Part model, mm, in its own coordinate system. Face numbers are marked on the shaded views. Give positions to 0.01 mm unless a question says otherwise; leave off trailing zeros. Write each loop counter-clockwise with the first axis right and the second up, starting at its lowest first coordinate (ties: lowest second). Pieces come first, ordered by that corner, then holes. Notation, with made-up numbers: M 60,62.25 L 103,62.25 A17 ccw 103,92.25 Z; hole C 22.25,60.25 d6. An arc over 180 degrees is marked long. Use a Markdown table: item, result. Add a question column.
from build123d import *

# Parameters (mm, degrees)
SKETCH1_R           = 4.5
BOSS_EXTRUDE1_DEPTH = 3
FILLET1_R           = 1
SKETCH6_R           = 1.75
BOSS_EXTRUDE3_DEPTH = 14
BOSS_EXTRUDE4_DEPTH = 1


with BuildPart() as part:
    # Sketch1 → Boss-Extrude1 (new body)
    with BuildSketch(Plane(origin=(0, 115.601531763, -5.053e-06), x_dir=(1, 0, 0), z_dir=(0, 1, -4.4e-08))):
        with Locations((40.91030477, -143.155151275)):
            Circle(SKETCH1_R)
    extrude(amount=BOSS_EXTRUDE1_DEPTH)

    # Fillet1
    fillet1_edges = [part.edges().sort_by_distance(p)[0] for p in [
        (36.41030477, 118.601538021, 143.155146091),
    ]]
    fillet(fillet1_edges, radius=FILLET1_R)

    # Sketch6 → Boss-Extrude3 (add)
    with BuildSketch(Plane(origin=(0, 115.601531763, -5.053e-06), x_dir=(-1, 0, 0), z_dir=(0, -1, 4.4e-08))):
        with Locations((-40.91030477, -143.155151275)):
            Circle(SKETCH6_R)
    extrude(amount=BOSS_EXTRUDE3_DEPTH)

    # Sketch7 → Boss-Extrude4 (add)
    with BuildSketch(Plane(origin=(0, 118.601531763, -5.184e-06), x_dir=(1, 0, 0), z_dir=(0, 1, -4.4e-08))):
        with BuildLine():
            add(Edge.make_bspline(
                [(39.781937709, -141.764742389), (39.830929551, -141.76598327), (39.927153571, -141.768420461), (40.068573285, -141.787076688), (40.203582672, -141.81935237), (40.333281527, -141.862338077), (40.45611848, -141.91968038), (40.573018119, -141.988989986), (40.683702303, -142.070993023), (40.786679181, -142.165055594), (40.880913899, -142.267399038), (40.96393704, -142.376617458), (41.033516631, -142.492050481), (41.090655886, -142.613351228), (41.135482812, -142.740245371), (41.16641566, -142.873409408), (41.186174857, -143.011980537), (41.188484879, -143.106494893), (41.189656726, -143.154440907)],
                knots=[0, 0, 0, 0, 0.000146952, 0.000288625, 0.000426954, 0.000562883, 0.000697813, 0.000832796, 0.000969967, 0.001110296, 0.00125059, 0.001386805, 0.001521151, 0.001654161, 0.00178843, 0.001924058, 0.002063701, 0.002207476, 0.002207476, 0.002207476, 0.002207476], degree=3))
            add(Edge.make_bspline(
                [(41.189656726, -143.154440907), (41.188485051, -143.202033739), (41.186175543, -143.295844723), (41.166393194, -143.433536493), (41.135368152, -143.565896722), (41.091072165, -143.692704448), (41.034205286, -143.814093439), (40.964162388, -143.929744292), (40.88165683, -144.039694918), (40.787762365, -144.142740802), (40.685405625, -144.237232938), (40.575618459, -144.319570421), (40.460869938, -144.390421396), (40.339683432, -144.446954293), (40.213666142, -144.492139018), (40.08169022, -144.522946066), (39.944374075, -144.542817819), (39.850733494, -144.545099673), (39.803138297, -144.546259483)],
                knots=[0, 0, 0, 0, 0.000142716, 0.000281309, 0.000416421, 0.000550016, 0.000683505, 0.000817851, 0.000954912, 0.001095241, 0.001235536, 0.001372174, 0.001506342, 0.001639351, 0.001772621, 0.001907218, 0.002045287, 0.002188002, 0.002188002, 0.002188002, 0.002188002], degree=3))
            add(Edge.make_bspline(
                [(39.803138297, -144.546259483), (39.755192532, -144.545088221), (39.660678666, -144.54277935), (39.521933407, -144.522987455), (39.388675827, -144.492037779), (39.261287002, -144.447807431), (39.139695894, -144.390644406), (39.023664701, -144.320942286), (38.913659155, -144.238235697), (38.810591287, -144.144371679), (38.716286834, -144.042188423), (38.634069925, -143.932700623), (38.564352131, -143.818056319), (38.50738104, -143.697937357), (38.46227755, -143.572924422), (38.431506646, -143.442183608), (38.41159792, -143.306460291), (38.409303721, -143.214050481), (38.408139632, -143.16716126)],
                knots=[0, 0, 0, 0, 0.000143775, 0.000283418, 0.000419562, 0.000553657, 0.000687146, 0.000821946, 0.000959007, 0.001099336, 0.001239631, 0.001375527, 0.001509419, 0.001641471, 0.001773742, 0.001907308, 0.002043802, 0.0021844, 0.0021844, 0.0021844, 0.0021844], degree=3))
            add(Edge.make_bspline(
                [(38.408139632, -143.16716126), (38.408543791, -143.135688944), (38.40934701, -143.073141351), (38.419016921, -142.980260052), (38.433048683, -142.888872471), (38.453158462, -142.799238481), (38.479459306, -142.711577499), (38.510492683, -142.625284958), (38.548396019, -142.541235357), (38.59124389, -142.459030531), (38.639066804, -142.379951936), (38.691889543, -142.305203679), (38.747856756, -142.234158521), (38.809212417, -142.168657512), (38.873934373, -142.106795165), (38.943072551, -142.049522158), (39.016205081, -141.996322047), (39.093646642, -141.948379289), (39.173489029, -141.905018514), (39.255794688, -141.867809139), (39.339445787, -141.835873128), (39.424834122, -141.809988695), (39.511732943, -141.789553763), (39.600331912, -141.77563868), (39.690560442, -141.765944106), (39.75134757, -141.765144685), (39.781937709, -141.764742389)],
                knots=[0, 0, 0, 0, 9.438e-05, 0.000187569, 0.000279848, 0.000371657, 0.000462884, 0.000554264, 0.000646556, 0.00073925, 0.000832238, 0.000923551, 0.001013693, 0.001103328, 0.001192553, 0.001282131, 0.001372457, 0.00146364, 0.001555178, 0.001644836, 0.001734413, 0.00182361, 0.001912319, 0.002001981, 0.002092533, 0.002184264, 0.002184264, 0.002184264, 0.002184264], degree=3))
        make_face()
        with BuildLine():
            add(Edge.make_bspline(
                [(39.793598032, -142.036109911), (39.768489351, -142.036415989), (39.718512029, -142.037025218), (39.6442136, -142.045050193), (39.570892316, -142.056487669), (39.498533037, -142.072802271), (39.42743852, -142.095030335), (39.356946081, -142.12061245), (39.287698534, -142.151773631), (39.219924487, -142.186980378), (39.154220829, -142.225948908), (39.092223132, -142.269016851), (39.033770895, -142.31517421), (38.979007235, -142.364528706), (38.928092956, -142.417331679), (38.88002595, -142.472782628), (38.836732873, -142.532466498), (38.797056276, -142.594764841), (38.761550826, -142.659596512), (38.729978206, -142.726278968), (38.704151843, -142.795356148), (38.683089213, -142.866078636), (38.665626856, -142.938334424), (38.654564306, -143.012671643), (38.646451153, -143.088716757), (38.645876746, -143.140107802), (38.645586213, -143.16610123)],
                knots=[0, 0, 0, 0, 7.5292e-05, 0.000149864, 0.00022393, 0.000297861, 0.000372133, 0.000447257, 0.000522705, 0.000599749, 0.000676284, 0.000751707, 0.000826039, 0.000899591, 0.000972681, 0.001045978, 0.001119549, 0.001193655, 0.001267426, 0.001341167, 0.0014148, 0.001488412, 0.001562462, 0.001637575, 0.001713729, 0.00179167, 0.00179167, 0.00179167, 0.00179167], degree=3))
            add(Edge.make_bspline(
                [(38.645586213, -143.16610123), (38.646549948, -143.204323861), (38.648445913, -143.279519602), (38.66504479, -143.389713377), (38.690612592, -143.495613451), (38.728302387, -143.59664037), (38.775436483, -143.693662536), (38.833665144, -143.785819258), (38.902652667, -143.873135443), (38.981017357, -143.95500151), (39.066683927, -144.029724231), (39.15764974, -144.095313236), (39.252940265, -144.150807889), (39.352803996, -144.196017676), (39.45670779, -144.231842061), (39.565321177, -144.25639436), (39.677920631, -144.272553186), (39.754672972, -144.274104972), (39.793598032, -144.274891962)],
                knots=[0, 0, 0, 0, 0.000114606, 0.000225465, 0.000333574, 0.000440894, 0.000548272, 0.000656647, 0.000767237, 0.000881574, 0.000996152, 0.001107795, 0.001217519, 0.00132639, 0.001436175, 0.001546614, 0.001660023, 0.001776724, 0.001776724, 0.001776724, 0.001776724], degree=3))
            add(Edge.make_bspline(
                [(39.793598032, -144.274891962), (39.819761167, -144.274532503), (39.871650522, -144.273819589), (39.948829875, -144.266639042), (40.024618797, -144.255124474), (40.098910985, -144.238545942), (40.171622122, -144.217797161), (40.243055694, -144.193147272), (40.31245083, -144.162394219), (40.380682969, -144.128415708), (40.445994414, -144.089680589), (40.508341989, -144.048074369), (40.566154188, -144.001984995), (40.620876879, -143.953363791), (40.672000191, -143.901230406), (40.719178411, -143.845652619), (40.762252678, -143.786279622), (40.801914208, -143.724075774), (40.837295246, -143.659066702), (40.868122303, -143.592142481), (40.89427532, -143.523467905), (40.915387939, -143.452943919), (40.931932306, -143.380704468), (40.943332007, -143.306652825), (40.951306125, -143.230937132), (40.951907165, -143.179726003), (40.952210145, -143.153910892)],
                knots=[0, 0, 0, 0, 7.8471e-05, 0.000155631, 0.000232315, 0.000308314, 0.000383811, 0.000459075, 0.000534795, 0.000611356, 0.000687621, 0.000762445, 0.000836033, 0.000909231, 0.000981942, 0.001054895, 0.001127725, 0.001201831, 0.001276067, 0.001349584, 0.001422723, 0.001496334, 0.001570264, 0.001644854, 0.001721008, 0.001798419, 0.001798419, 0.001798419, 0.001798419], degree=3))
            add(Edge.make_bspline(
                [(40.952210145, -143.153910892), (40.951906923, -143.128272386), (40.951305425, -143.077413686), (40.943335816, -143.002226044), (40.931920262, -142.928707247), (40.915468691, -142.85714592), (40.894264111, -142.787523821), (40.868117736, -142.719906339), (40.837285992, -142.654041572), (40.801901203, -142.590092312), (40.762126146, -142.528728075), (40.718663236, -142.470064347), (40.67076205, -142.41520281), (40.619791186, -142.362789083), (40.564477481, -142.313941036), (40.505071497, -142.268642464), (40.442294431, -142.225800167), (40.375825628, -142.187151677), (40.30722752, -142.151459965), (40.236837802, -142.120880933), (40.165453899, -142.094897248), (40.093257338, -142.072735018), (40.019640444, -142.056551567), (39.945100645, -142.045039886), (39.869741068, -142.037028011), (39.819059587, -142.036416915), (39.793598032, -142.036109911)],
                knots=[0, 0, 0, 0, 7.6881e-05, 0.000152508, 0.000226574, 0.000299988, 0.000372585, 0.000444733, 0.000517289, 0.000590596, 0.000663809, 0.000736527, 0.000809423, 0.000882134, 0.000955727, 0.00103057, 0.00110613, 0.001183578, 0.001261092, 0.001337996, 0.001413617, 0.001488903, 0.001564385, 0.001639498, 0.001715125, 0.001791477, 0.001791477, 0.001791477, 0.001791477], degree=3))
        make_face(mode=Mode.SUBTRACT)
        Polygon((41.732391769, -141.83258427), (41.96983835, -141.83258427), (41.96983835, -142.840142196), (43.07279892, -141.83258427), (43.411478307, -141.83258427), (42.111352272, -143.019817176), (43.513241128, -144.478417603), (43.196822358, -144.478417603), (41.96983835, -143.201612214), (41.96983835, -144.478417603), (41.732391769, -144.478417603), align=None)
    extrude(amount=BOSS_EXTRUDE4_DEPTH)


solid = part.part
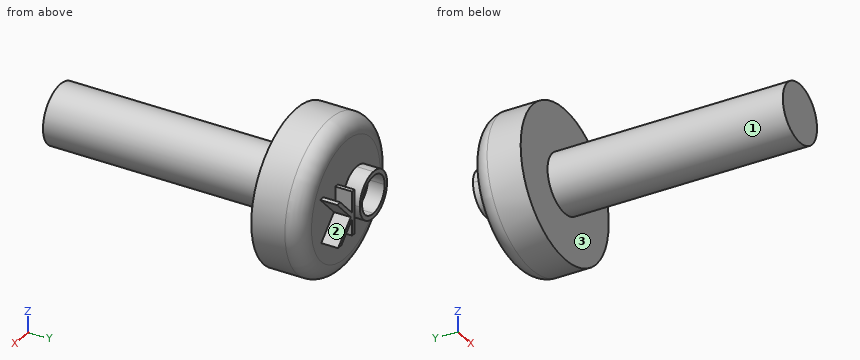
1. Drill centre lines: probe 1 along Y at (x, z) = (40.25, 145.5); probe 2 along Y at (x, z) = (41.5, 142); probe 3 along X at (y, z) = (112, 143). Where is each one in solid material? Low to high. Write a range as [from, to].
2. Cut at A-A (y = 110.75). Write the cut outline in (x, z).
3. Flat gauge pins, fed straight in: pin 1 (5 mm diameter, centred on x = 38, y = 112.5, fed in from -Z); pin 2 (5 mm diameter, centred on x = 41, z = 141, fed in from -Y); pin 3 (5 mm diameter, centred on y = 107.5, z = 141, fed in from +X); pin 4 (0.7 mm diameter, centred on x = 40, z = 143.5, fed in from +Y). Where does each tip first touch, or does it go through?
4. Mould opens along Z. For the marked faces 1, 2 and 3 say: released by +Z, released by -Z, zero draft, split by the parting line, or undercut.
A:
| question | item | result |
|---|---|---|
| 1 | probe 1 | y = [115.6, 118.6] |
| 1 | probe 2 | y = [101.6, 118.6] |
| 1 | probe 3 | x = [39.17, 42.65] |
| 2 | outline | C 40.91,143.16 d3.5 |
| 3 | pin 1 | stops at z = 141.45 |
| 3 | pin 2 | stops at y = 101.6 |
| 3 | pin 3 | stops at x = 42.66 |
| 3 | pin 4 | stops at y = 118.6 |
| 4 | face 1 | split by the parting line |
| 4 | face 2 | undercut |
| 4 | face 3 | zero draft |
